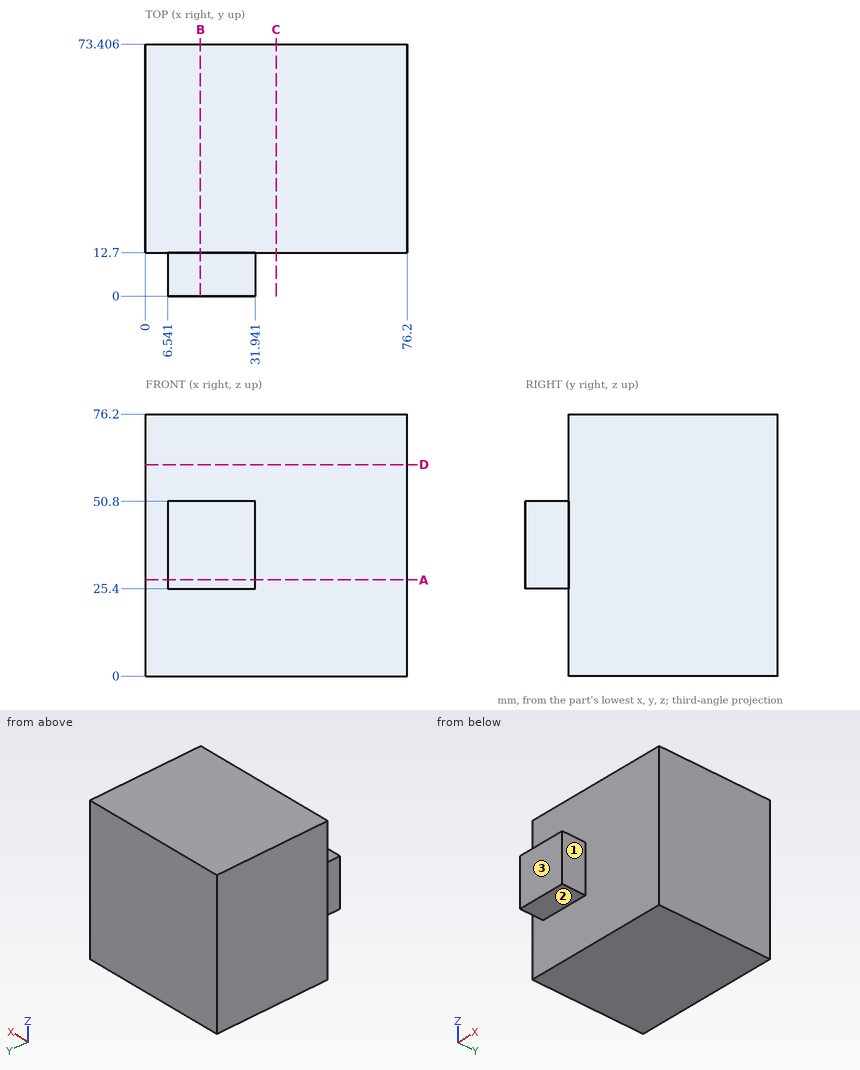
Answer from the drawing. Dimensions are ordinates in mm from the lowest x, y and z of the part. A direction names the side the tool comes from. Coordinates: 2 decimals unless noted, no trailing zeros. Order: outer loops, then holes, each group sorted by start corner. A loop starts at its lowest first (then second) coordinate and runs counter-clockwise, first axis right, second up. Notation, with made-up numbers: (0, 86) - (5, 86) arc R21 cw to (5, 112) - close; hole circle Ø7 at (51, 85). An arc over 180 degrees is marked (long way). Answer as a JSON object with one key per item and string values. Group by question number.
Item 1: Section B-B (x = 16) is taken. Give the vertices of the cut face in (y, z).
Item 2: Section D-D (z = 61.5) is taken. Give the vertices of the cut face in (x, y), plus the area to 3 significant figures.
Item 3: Section A-A (z = 28) is taken. Give the vertices of the cut face in (x, y).
Item 4: Flat-ended cylindrical pins translate along their axes: P1, Ø14, axis at x = 16, y = 3.5, coming from the -Z side; P2, Ø4, axis at x = 50.5, z = 62, coming from the -Y side; P3, Ø6.5, axis at x = 17.5, y = 6.5, coming from the +Z side; P4, Ø6, axis at y = 7.5, z = 56.5, coming from the +X side. Find the tip coordinate at first contact, or state that the pin passes through.
Item 5: A tool of negligible diameter and unlimited length cuts with its end or side. For the marked faces 1, 2 and 3, from which of +Z, -Z, +X, -X, +Y, -Y can it reach the whole face along a straight path? Write none if from no direction.
Item 6: Section C-C (x = 38) is taken. Give the vertices of the cut face in (y, z), plus the area to 3 significant figures.
Item 7: Consider probe 1 along Y at (x, z) = (5, 26). Determine where the line is inside the solid, lowest interval first. Write a range as from..to.
Results are:
{
 "1": {"outline": "(0, 25.4) - (12.7, 25.4) - (12.7, 0) - (73.41, 0) - (73.41, 76.2) - (12.7, 76.2) - (12.7, 50.8) - (0, 50.8) - close"},
 "2": {"outline": "(0, 12.7) - (76.2, 12.7) - (76.2, 73.41) - (0, 73.41) - close", "area": "4,630 mm^2"},
 "3": {"outline": "(0, 12.7) - (6.54, 12.7) - (6.54, 0) - (31.94, 0) - (31.94, 12.7) - (76.2, 12.7) - (76.2, 73.41) - (0, 73.41) - close"},
 "4": {"P1": "stops at z = 25.4", "P2": "stops at y = 12.7", "P3": "stops at z = 50.8", "P4": "passes through"},
 "5": {"face 1": "+Z, -Z, +X, -Y", "face 2": "-Z, +X, -X, -Y", "face 3": "+Z, -Z, +X, -X, -Y"},
 "6": {"outline": "(12.7, 0) - (73.41, 0) - (73.41, 76.2) - (12.7, 76.2) - close", "area": "4,630 mm^2"},
 "7": {"probe 1": "y = 12.7..73.41"}
}
